Here's how the part is built. I have some questions about the finished solid (model axes, mm). Face numbers are marked on the shaded views. Give positions to 0.01 mm unless a question says otherwise; leave off trailing zeros.
Q1. Suppose I cut it at A-A (y = 10.5). Count the separate pieces of the cut face and the enclosed holes in it, and give its area (3 significant figures).
Q2. Thinking about a two-plate mould opening in Y: for the marked faces 1 and 2, which applies, pulls with the +Y half, pulls with the -Y half, needs draft (parallel to the pull), parting line crosses it, or undercut?
Q3. I need wall thicknesses on probe 1 along Z at (x, y) = (-18, 14.25); probe 2 along Z at (x, y) = (-123, 8.25); probe 3 along X at (y, z) = (4.5, -31). Which ranges of each line are inside material? Lowest first, please.
Q4. I'm going to push flat-ended pins straight in: P1, Ø5, axis at x = -160.53, z = 19.43, coming from the -Y side; P2, Ø4.5, axis at y = 6.5, z = 68, coming from the -X side. Where does each tip first touch, or does it pass through?
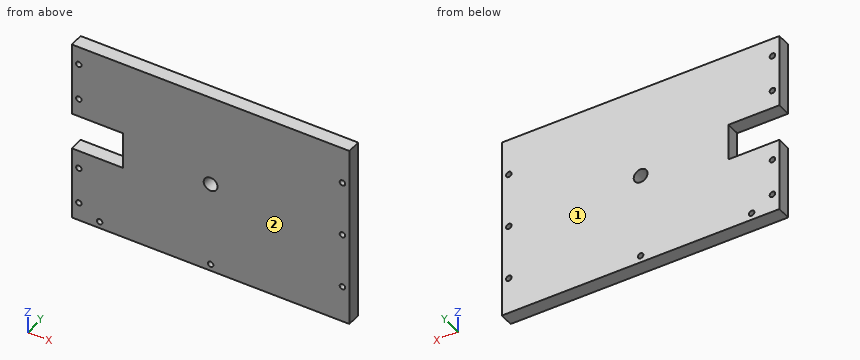
```python
from build123d import *

# Parameters (mm, degrees)
SKETCH2_R           = 7.5
SKETCH2_R_2         = 3
BOSS_EXTRUDE2_DEPTH = 15


with BuildPart() as part:
    # Sketch2 → Boss-Extrude2 (new body)
    with BuildSketch(Plane(origin=(0, 0, 0), x_dir=(1, 0, 0), z_dir=(0, 1, 0))):
        Polygon((-168.032786885, 40.573770492), (131.967213115, 40.573770492), (131.967213115, -159.426229508), (-168.032786885, -159.426229508), (-168.032786885, -79.426229508), (-113.032786885, -79.426229508), (-113.032786885, -39.426229508), (-168.032786885, -39.426229508), align=None)
        with Locations(Location((-18.032786885, -59.426229508, 0), (0, 0, 270))):
            Circle(SKETCH2_R, mode=Mode.SUBTRACT)
        with Locations(Location((-160.532786885, 20.573770492, 0), (0, 0, 270))):
            Circle(SKETCH2_R_2, mode=Mode.SUBTRACT)
        with Locations(Location((-160.532786885, -19.426229508, 0), (0, 0, 90))):
            Circle(SKETCH2_R_2, mode=Mode.SUBTRACT)
        with Locations(Location((-160.532786885, -139.426229508, 0), (0, 0, 270))):
            Circle(SKETCH2_R_2, mode=Mode.SUBTRACT)
        with Locations(Location((-160.532786885, -99.426229508, 0), (0, 0, 90))):
            Circle(SKETCH2_R_2, mode=Mode.SUBTRACT)
        with Locations(Location((124.467213115, -119.426229508, 0), (0, 0, 270))):
            Circle(SKETCH2_R_2, mode=Mode.SUBTRACT)
        with Locations(Location((124.467213115, 0.573770492, 0), (0, 0, 90))):
            Circle(SKETCH2_R_2, mode=Mode.SUBTRACT)
        with Locations(Location((124.467213115, -59.426229508, 0), (0, 0, 270))):
            Circle(SKETCH2_R_2, mode=Mode.SUBTRACT)
        with Locations(Location((-18.032786885, 33.073770492, 0), (0, 0, 270))):
            Circle(SKETCH2_R_2, mode=Mode.SUBTRACT)
        with Locations(Location((-138.032786885, 33.073770492, 0), (0, 0, 270))):
            Circle(SKETCH2_R_2, mode=Mode.SUBTRACT)
    extrude(amount=BOSS_EXTRUDE2_DEPTH)


solid = part.part
```
Solutions:
1. separate pieces: 1
1. enclosed holes: 10
1. area: 57,400 mm2
2. face 1: pulls with the +Y half
2. face 2: pulls with the -Y half
3. probe 1: z = -40.57 to -36.07, -30.07 to 51.93, 66.93 to 159.43
3. probe 2: z = -40.57 to 39.43, 79.43 to 159.43
3. probe 3: x = -168.03 to -140.2, -135.86 to -20.2, -15.86 to 131.97
4. P1: passes through
4. P2: stops at x = -113.03
